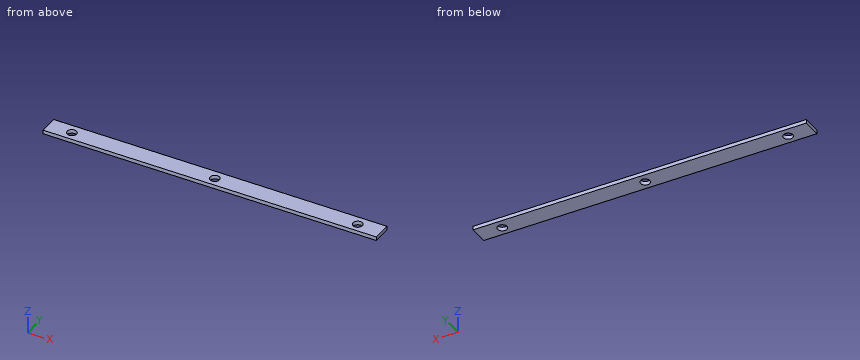
```python
from build123d import *

# Parameters (mm, degrees)
SKETCH1_W                    = 177.8
SKETCH1_H                    = 10
BOSS_EXTRUDE1_DEPTH          = 2
F_5_0_5_DIAMETER_HOLE1_D     = 5
F_5_0_5_DIAMETER_HOLE1_DEPTH = 5
F_5_0_5_DIAMETER_HOLE1_TIP   = 1.502151548


with BuildPart() as part:
    # Sketch1 → Boss-Extrude1 (new body)
    with BuildSketch(Plane.XY):
        with Locations((43.423133199, 0.190336281)):
            Rectangle(SKETCH1_W, SKETCH1_H)
    extrude(amount=BOSS_EXTRUDE1_DEPTH)

    # Ø5.0 (5) Diameter Hole1
    with Locations(Plane.XY.offset(2)):
        with Locations((-32.776866801, 0), (43.423133199, 0), (119.623133199, 0)):
            Hole(F_5_0_5_DIAMETER_HOLE1_D / 2, depth=F_5_0_5_DIAMETER_HOLE1_DEPTH)
            with Locations((0, 0, -(F_5_0_5_DIAMETER_HOLE1_DEPTH + F_5_0_5_DIAMETER_HOLE1_TIP / 2))):  # 118° drill point
                Cone(0, F_5_0_5_DIAMETER_HOLE1_D / 2, F_5_0_5_DIAMETER_HOLE1_TIP, mode=Mode.SUBTRACT)


solid = part.part
```
Work out the finished part from the listing and answer in its coordinate system (mm). Give positions to 0.01 mm unless a question says otherwise; leave off trailing zeros. Write each loop counter-clockwise with the first axis right and the second up, starting at its lowest first coordinate (ties: lowest second). Pieces come first, ordered by that corner, then holes. Notation, with made-up numbers: (-2, 78) -> (48, 78) arc R24 cw to (48, 115) -> close; hole circle Ø7 at (-36.5, -40). An arc over 180 degrees is marked (long way). Write item = value, one per line.
Q1. Section B-B on z = 1.25 is taken. Determine the outline of the cut face in (x, y).
Computed values:
outline = (-45.48, -4.81) -> (132.32, -4.81) -> (132.32, 5.19) -> (-45.48, 5.19) -> close; hole circle Ø5 at (-32.78, 0); hole circle Ø5 at (43.42, 0); hole circle Ø5 at (119.62, 0)
Q2. Consider line 1 along X through (y, z) = (1.75, 1.25); line 2 along X through (y, z) = (0.75, 1.3); line 3 along Y through (x, z) = (42.5, 0.7). Determine where each line is inside the solid, lowest interval first.
Computed values:
line_1 = -45.48 to -34.56, -30.99 to 41.64, 45.21 to 117.84, 121.41 to 132.32
line_2 = -45.48 to -35.16, -30.39 to 41.04, 45.81 to 117.24, 122.01 to 132.32
line_3 = -4.81 to -2.32, 2.32 to 5.19
Q3. Section A-A on y = 0 is taken. Determine the outline of the cut face in (x, z), and give its area (3 significant figures).
Computed values:
outline = (-45.48, 0) -> (-35.28, 0) -> (-35.28, 2) -> (-45.48, 2) -> close; (-30.28, 0) -> (40.92, 0) -> (40.92, 2) -> (-30.28, 2) -> close; (45.92, 0) -> (117.12, 0) -> (117.12, 2) -> (45.92, 2) -> close; (122.12, 0) -> (132.32, 0) -> (132.32, 2) -> (122.12, 2) -> close
area = 326 mm^2
